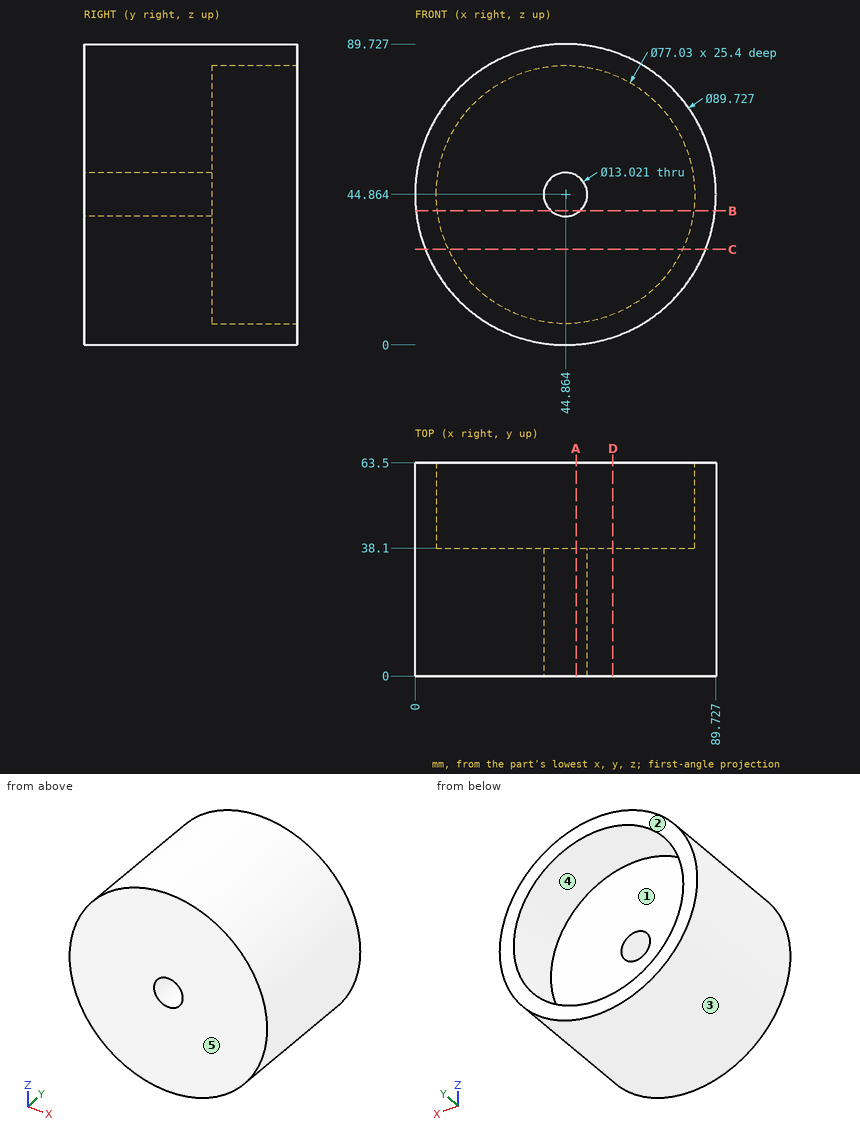
Input: dimensioned drawing with shaded views. Units: mm. Origin: part minimum x, y, z. A direction names the side the tool comes from. Coordinates: 2 decimals unless noted, no trailing zeros. Loops run counter-clockwise (first coordinate to the right, second up) from the corner with the lowest first, then second, coordinate; pieces in that order, holes last. Notation, with made-up numbers: M 30,-14.75 L 37,-14.75 A12 ccw 37,-0.75 Z; hole C 26.5,69 d5. An arc over 180 degrees is marked long. Put each result on its own line as item: value.
(1) Access query for the marked faces 1 and 2. Directions: +Z, -Z, +X, -X, +Y, -Y. A direction counts if a zero-diameter tool reaches every point of the face in a straight line with its end or side. Return the directions, or none.
Answer sheet:
face 1: +Y
face 2: +Z, -Z, +X, -X, +Y
(2) Cut plane A-A on x = 48. Return the cut outline in (y, z).
Answer sheet:
outline: M 0,0.11 L 63.5,0.11 L 63.5,6.48 L 38.1,6.48 L 38.1,39.16 L 0,39.16 Z; M 0,50.57 L 38.1,50.57 L 38.1,83.25 L 63.5,83.25 L 63.5,89.62 L 0,89.62 Z
(3) Cut plane D-D on x = 59. Return the cut outline in (y, z) (1 decimal), then the cut area to 3 significant figures.
Answer sheet:
outline: M 0,2.3 L 63.5,2.3 L 63.5,9 L 38.1,9 L 38.1,80.7 L 63.5,80.7 L 63.5,87.4 L 0,87.4 Z
area: 3,590 mm^2
(4) First-contact query: pin 1 (4 mm diameter, centred on x = 29.5, z = 13.5, fed in from +Y); pin 2 (12 mm diameter, centred on x = 68, y = 47, fed in from -Z); pin 3 (2 mm diameter, centred on x = 16.5, y = 24.5, fed in from +Z) (1 decimal). Flat tips, straight axial feed; report the tip coordinate or a pass-through.
Answer sheet:
pin 1: stops at y = 38.1
pin 2: stops at z = 3.4
pin 3: stops at z = 80.4
(5) Cut plane C-C on z = 28.5. Return the cut outline in (x, y), then the cut area to 3 significant figures.
Answer sheet:
outline: M 3.09,0 L 86.64,0 L 86.64,63.5 L 79.73,63.5 L 79.73,38.1 L 10,38.1 L 10,63.5 L 3.09,63.5 Z
area: 3,530 mm^2
(6) Draft query along Z for the marked faces 3, 4 and 5. Return one class per face: pulls with the +Z half, pulls with the -Z half, needs draft (parallel to the pull), parting line crosses it, or undercut.
Answer sheet:
face 3: parting line crosses it
face 4: undercut
face 5: needs draft
(7) Cut plane B-B on z = 40. Return the cut outline in (x, y) (1 decimal), then the cut area to 3 significant figures.
Answer sheet:
outline: M 0.3,0 L 40.5,0 L 40.5,38.1 L 6.7,38.1 L 6.7,63.5 L 0.3,63.5 Z; M 49.2,0 L 89.5,0 L 89.5,63.5 L 83.1,63.5 L 83.1,38.1 L 49.2,38.1 Z
area: 3,390 mm^2
(8) Material intervals for probe 1 along Y at (x, z) = (54.5, 58); probe 2 along Z at (x, y) = (34, 46.5) (1 decimal); probe 3 along Z at (x, y) = (22, 58) (1 decimal), sorted ascending.
Answer sheet:
probe 1: y = 0 to 38.1
probe 2: z = 1.3 to 7.9, 81.8 to 88.4
probe 3: z = 6.3 to 13.9, 75.9 to 83.5
